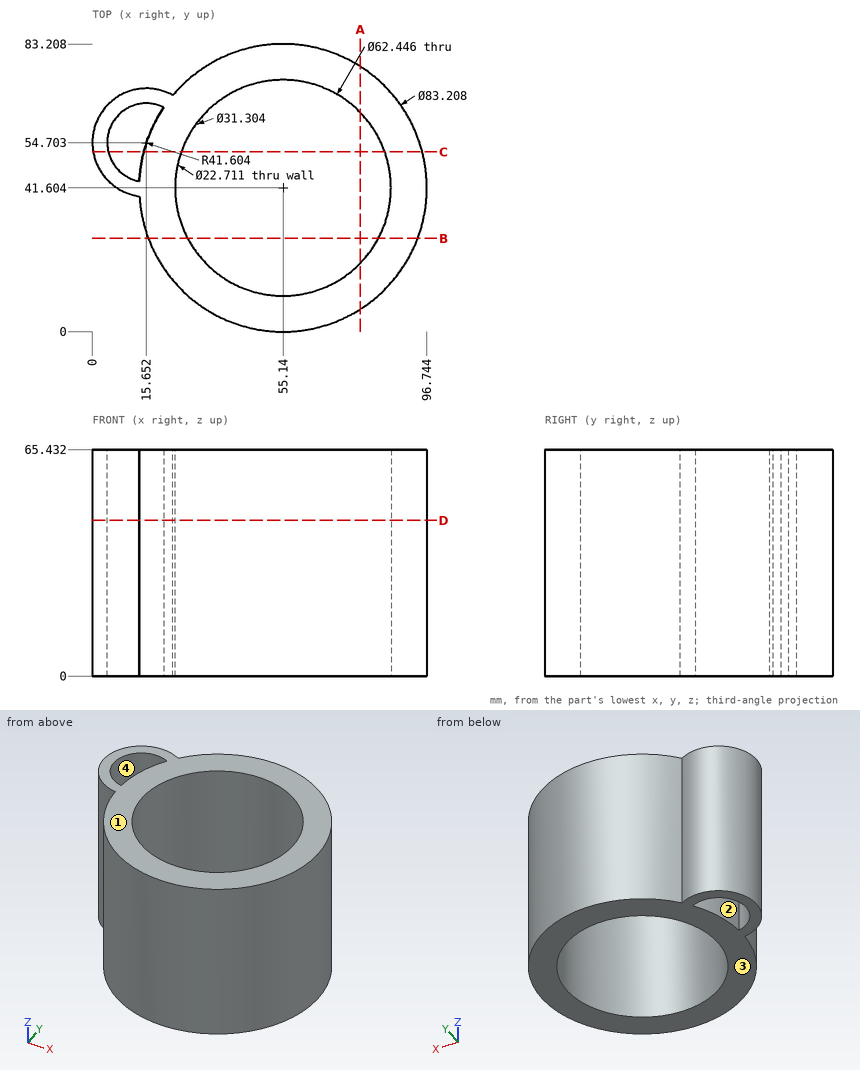
Study the drawing (mm; zero at the part's minimum x, y, z) and answer. A direction names the side the tool comes from. Round coordinates to 2 decimals unless told otherwise and drop trailing zeros. Order: outer loops, then holes, each group sorted by start corner. A loop starts at its lowest first (then second) coordinate and runs counter-clockwise, first axis right, second up. Notation, with made-up numbers: M 71.5,38.5 L 118.5,38.5 A19 ccw 118.5,45.5 Z; hole C 9.5,5.5 d7. An arc over 180 degrees is marked long. One line per item, written item: value.
Q1. For the marked faces 1 and 2, determine the directions among +Z, -Z, +X, -X, +Y, -Y from which every point of the face is accessible in a straight line to the end or side of a thin tool.
Derived:
face 1: +Z, +X, -X, +Y, -Y
face 2: +Z, -Z
Q2. Find section A-A on x = 77.5. Write down the section's boundary in (y, z).
Derived:
outline: M 6.52,0 L 19.81,0 L 19.81,65.43 L 6.52,65.43 Z; M 63.4,0 L 76.69,0 L 76.69,65.43 L 63.4,65.43 Z
Q3. Find section D-D on z = 45. Write down the section's boundary in (x, y) (1 decimal), then the cut area to 3 significant figures.
Derived:
outline: M 13.6,39.2 A41.6 ccw long 23.3,68.4 A15.7 ccw long Z; hole M 13.6,43.5 A41.6 cw 20.7,64.9 A11.4 ccw long Z; hole C 55.1,41.6 d62.4
area: 2,580 mm²
Q4. Find section C-C on y = 52. Write down the section's boundary in (x, z) (1 decimal).
Derived:
outline: M 0.2,0 L 4.6,0 L 4.6,65.4 L 0.2,65.4 Z; M 14.9,0 L 25.7,0 L 25.7,65.4 L 14.9,65.4 Z; M 84.6,0 L 95.4,0 L 95.4,65.4 L 84.6,65.4 Z
Q5. Determine the mould class of the marked faces 3 and 4 for opening direction X: released by +X, released by -X, zero draft, split by the parting line, or undercut.
Derived:
face 3: zero draft
face 4: undercut
Q6. Find section B-B on y = 27. Write down the section's boundary in (x, z).
Derived:
outline: M 16.18,0 L 27.54,0 L 27.54,65.43 L 16.18,65.43 Z; M 82.74,0 L 94.1,0 L 94.1,65.43 L 82.74,65.43 Z
Q7. Straight lines are drawn through the part: line 1 (X direction, y = 54, z = 5.5) (1 decimal); line 2 (X direction, y = 52, z = 52) (1 decimal); line 3 (Y direction, x = 54.5, z = 4.5) (1 decimal). For each, find the intervals that lie inside material, in ascending order.
Derived:
line 1: 0 to 4.3, 15.4 to 26.5, 83.8 to 94.9
line 2: 0.2 to 4.6, 14.9 to 25.7, 84.6 to 95.4
line 3: 0 to 10.4, 72.8 to 83.2
Q8. Flat-ended cylindrical pins translate along their axes: pin 1 (4 mm diameter, centred on x = 15.5, z = 7, fed in from +Y) (1 decimal); pin 2 (3 mm diameter, centred on x = 10.5, z = 41.5, fed in from -Y); pin 3 (1.5 mm diameter, centred on y = 58.5, z = 32, fed in from -X). Find the tip coordinate at first contact, or state that the pin passes through.
Derived:
pin 1: y = 70.4
pin 2: y = 39.48
pin 3: x = 0.3
